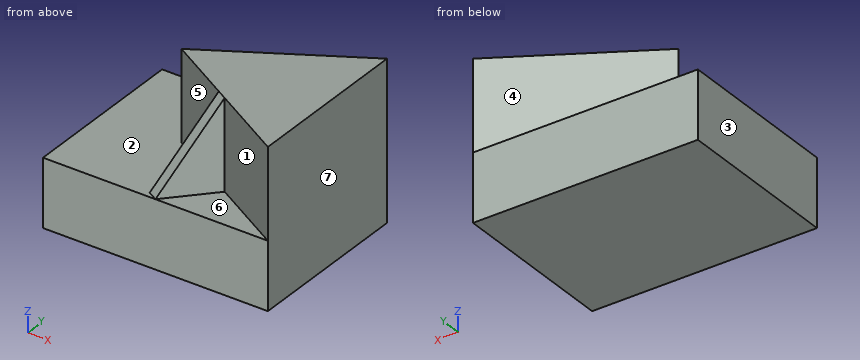
from build123d import *

# Parameters (mm, degrees)
SKETCH_1_W      = 20
SKETCH_1_H      = 15
EXTRUDE_1_DEPTH = 3
EXTRUDE_2_DEPTH = 8
EXTRUDE_3_DEPTH = 1


with BuildPart() as part:
    # Sketch 1 → Extrude 1 (new, symmetric)
    with BuildSketch(Plane.XY):
        with Locations((-7.014925373, 7.5)):
            Rectangle(SKETCH_1_W, SKETCH_1_H)
    extrude(amount=EXTRUDE_1_DEPTH, both=True)



with BuildPart() as body_2:
    # Sketch 2 → Extrude 2 (new body)
    with BuildSketch(Plane.XY.offset(3)):
        Polygon((2.985074627, 0), (2.985074627, 15), (-10.00530643, 7.5), align=None)
    extrude(amount=EXTRUDE_2_DEPTH)


with BuildPart() as part_1:
    add(part.part)

    add(body_2.part)  # Extrude 3 merges body 2
    # Sketch 3D_1 → Extrude 3 (add, along a direction that is not the sketch's normal)
    with BuildSketch(Plane(origin=(-3.510115902, 3.75, 11), x_dir=(-0.368730866446014, -0.3945266526955367, -0.8416568590838117), z_dir=(0.7305877107722233, -0.6828188609496683, 0))):
        Polygon((0, 0), (9.505061253, 0), (6.733254873, 4.320101714), align=None)
    extrude(amount=-EXTRUDE_3_DEPTH, dir=(0.8660254037844387, -0.49999999999999983, 0))


solid = part_1.part
For this review, take the finished solid that the model builds, in its own axes (mm). Face numbers are marked on the shaded views. A direction names the side the tool comes from. Round coordinates to 2 decimals unless told otherwise and drop trailing zeros. Loops run counter-clockwise (first coordinate to the right, second up) from the corner with the lowest first, then second, coordinate; pieces in that order, holes last. Notation, with made-up numbers: (-9, 55) - (34, 55) arc R27 ccw to (34, 84) - close; hole circle Ø8 at (-7.75, 52.25). An arc over 180 degrees is marked (long way). Answer as CSV lines item,"result".
(1) Wall thickness on line 1 (Z direction, x = -15.75, y = 14); line 2 (Y direction, x = -6, z = 4); line 3 (X direction, y = 10.75, z = 5.25): over which ranges is each line inside the solid? List them lowest first.
Checked values:
line 1,"z = -3 to 3"
line 2,"y = 1.09 to 2.51, 5.19 to 9.81"
line 3,"x = -4.38 to 2.99"
(2) Insertion check: P1, Ø3, axis at x = -10.5, y = 5.5, coming from the +Z side; P2, Ø4, axis at x = -4.5, y = 1, coming from the +Z side. Each pin has a flat end and moves straight along its axis. Give the tip position at first contact, or say it passes through.
Checked values:
P1,"stops at z = 3"
P2,"stops at z = 9.36"
(3) Consider section D-D on z = 8.75. Give the boundary of the cut face in (x, y).
Checked values:
outline,"(-10.01, 7.5) - (-4.38, 4.25) - (-5.36, 3.2) - (-4.5, 2.7) - (-3.51, 3.75) - (2.99, 0) - (2.99, 15) - close"
(4) Consider section A-A on y = 11.25. Give the boundary of the cut face in (x, z).
Checked values:
outline,"(-17.01, -3) - (2.99, -3) - (2.99, 11) - (-3.51, 11) - (-3.51, 3) - (-17.01, 3) - close"
(5) Mouldability with a two-part tool opening along X and no side actions: class the marked faces 5, 6 and 7 as +X half, -X half, draft (parallel to the pull), parting line (faces both ways), or undercut.
Checked values:
face 5,"-X half"
face 6,"undercut"
face 7,"+X half"
(6) Consider section C-C on x = 1. Give the boundary of the cut face in (y, z).
Checked values:
outline,"(0, -3) - (15, -3) - (15, 3) - (13.85, 3) - (13.85, 11) - (1.15, 11) - (1.15, 3) - (0, 3) - close"
(7) Consider section B-B on z = 4. Give the boundary of the cut face in (x, y), then the cut area to 3 significant figures.
Checked values:
outline,"(-10.01, 7.5) - (-4.38, 4.25) - (-7.44, 0.97) - (-6.58, 0.47) - (-3.51, 3.75) - (2.99, 0) - (2.99, 15) - close"
area,"102 mm2"
(8) Tool access review of the marked faces 1, 2, 3 and 4: name each direction out of +Z, -Z, +X, -X, +Y, -Y from which nothing blocks a thin tool from reaching the whole face with its end or side.
Checked values:
face 1,"+Z, -Y"
face 2,"+Z, -X"
face 3,"+Z, -Z, -X, +Y, -Y"
face 4,"+Z, -X, +Y"
